Source: CAD feature listing. Evaluate the final solid. Frame: model axes, mm. Face numbers are marked on the shaded views. A direction names the side the tool comes from. Give positions to 0.01 mm unless a question says otherwise; leave off trailing zeros. Order: outer loops, then holes, each group sorted by start corner. A loop starts at its lowest first (then second) coordinate and runs counter-clockwise, first axis right, second up. Notation, with made-up numbers: M -39.5,32.25 L -3.5,32.25 A22 cw -3.5,49.25 Z; hole C 51,81 d9. An arc over 180 degrees is marked long. Return JSON: item names as keys, results as strings.
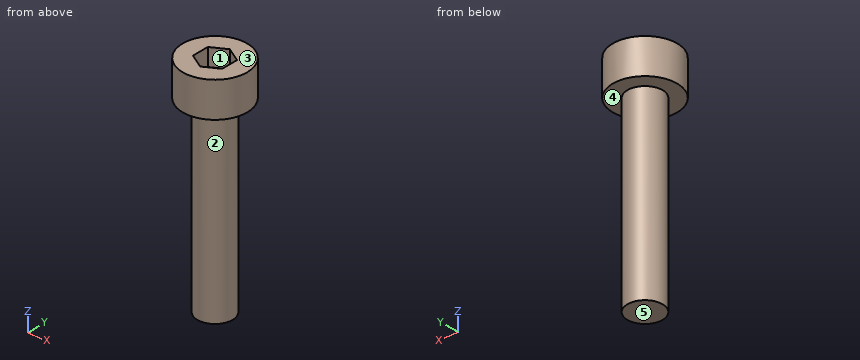
from build123d import *

# Parameters (mm, degrees)
SKETCH_1_R          = 2.75
EXTRUDE_1_DEPTH     = 3
CUT_EXTRUDE_1_DEPTH = 1.5
SKETCH_3_R          = 1.5
EXTRUDE_2_DEPTH     = 16


with BuildPart() as part:
    # 草图1 → 凸台-拉伸1 (new body)
    with BuildSketch(Plane.XY):
        Circle(SKETCH_1_R)
    extrude(amount=EXTRUDE_1_DEPTH)

    # 草图2 → 切除-拉伸1 (cut)
    with BuildSketch(Plane.XY.offset(3)):
        Polygon((0, -1.443375673), (1.25, -0.721687836), (1.25, 0.721687836), (0, 1.443375673), (-1.25, 0.721687836), (-1.25, -0.721687836), align=None)
    extrude(amount=-CUT_EXTRUDE_1_DEPTH, mode=Mode.SUBTRACT)

    # 草图3 → 凸台-拉伸2 (add)
    with BuildSketch(Plane(origin=(0, 0, 0), x_dir=(-1, 0, 0), z_dir=(0, 0, -1))):
        Circle(SKETCH_3_R)
    extrude(amount=EXTRUDE_2_DEPTH)


solid = part.part
1. Ray query, probe 1 along Z at (x, y) = (1, -1.6); probe 2 along Z at (x, y) = (0.9, 0.75); probe 3 along Y at (x, z) = (1, -10.25). Return the intervals inside material, ascending.
Evaluation:
{"probe 1": "z = 0 to 3", "probe 2": "z = -16 to 1.5", "probe 3": "y = -1.12 to 1.12"}
2. Section query A-A (y = 0). Return loops of the section in (x, z), then the cut area to 4 significant figures.
Evaluation:
{"outline": "M -2.75,0 L -1.5,0 L -1.5,-16 L 1.5,-16 L 1.5,0 L 2.75,0 L 2.75,3 L 1.25,3 L 1.25,1.5 L -1.25,1.5 L -1.25,3 L -2.75,3 Z", "area": "60.75 mm^2"}
3. Section query B-B (x = 0.6). Return loops of the section in (y, z), then the cut area to 3 significant figures.
Evaluation:
{"outline": "M -2.68,0 L -1.37,0 L -1.37,-16 L 1.37,-16 L 1.37,0 L 2.68,0 L 2.68,3 L 1.1,3 L 1.1,1.5 L -1.1,1.5 L -1.1,3 L -2.68,3 Z", "area": "56.8 mm^2"}
4. Draft query along X for the marked faces 1, 2 and 3. Return one class per face: pulls with the +X half, pulls with the -X half, needs draft (parallel to the pull), parting line crosses it, or undercut.
Evaluation:
{"face 1": "undercut", "face 2": "parting line crosses it", "face 3": "needs draft"}
5. Set-up query: the marked faces 4 and 5. Return all of +Z, -Z, +X, -X, +Y, -Y with unobstructed straight access to the full face (end or side cutting, diameter ignored); none if empty.
Evaluation:
{"face 4": "-Z", "face 5": "-Z, +X, -X, +Y, -Y"}
6. Section query C-C (z = -10.25). Return loops of the section in (x, y).
Evaluation:
{"outline": "C 0,0 d3"}
7. First-contact query: pin 1 (0.7 mm diameter, centred on y = -0.5, z = 2, fed in from +X). Flat tip, straight axial feed; report the tip coordinate or a pass-through.
Evaluation:
{"pin 1": "stops at x = 2.75"}
8. Section query D-D (x = -2.1). Return loops of the section in (y, z), then the cut area to 3 significant figures.
Evaluation:
{"outline": "M -1.78,0 L 1.78,0 L 1.78,3 L -1.78,3 Z", "area": "10.7 mm^2"}
